Autodesk Inventor part; units mm, degrees
ref_plane "YZ Plane" through (0, 0, 0) normal (1, 0, 0) x (0, 1, 0)
ref_plane "XZ Plane" through (0, 0, 0) normal (0, 1, 0) x (-1, 0, 0)
ref_plane "XY Plane" through (0, 0, 0) normal (0, 0, 1) x (1, 0, 0)
sketch "Sketch1" plane through (0, 0, 0) normal (0, 1, 0) x (-1, 0, 0)
  line L0 (0, 0) -> (-120, 0)
  line L1 (-120, 0) -> (-120, 70)
  line L2 (-120, 70) -> (0, 70)
  line L3 (0, 70) -> (0, 0)
  dimension "d0" = 120
  dimension "d1" = 70
extrude "Extrusion1" add sketch "Sketch1" along normal blind 1
sketch "Sketch2" plane through (0, 1, 0) normal (0, 1, 0) x (1, 0, 0)
  line L0 (120, -70) -> (120, 0)
  line L1 (120, 0) -> (0, 0)
  line L2 (120, -70) -> (90, -70)
  line L3 (90, -70) -> (90, 0)
  line L4 (90, 0) -> (120, 0)
  line L5 (120, 0) -> (120, -70)
  line L6 (0, 0) -> (0, -70)
  line L7 (0, -70) -> (90, -70)
  line L8 (90, -70) -> (90, -11)
  line L9 (90, -11) -> (0, -11)
  line L10 (0, -11) -> (0, -70)
  line L11 (0, 0) -> (84, 0)
  line L12 (84, 0) -> (84, -42)
  line L13 (84, -42) -> (0, -42)
  line L14 (0, -42) -> (0, 0)
  line L15 (0, 0) -> (6, 0)
  line L16 (6, 0) -> (6, -6)
  line L17 (6, -6) -> (0, -6)
  line L18 (0, -6) -> (0, 0)
  line L19 (84, 0) -> (78, 0)
  line L20 (78, 0) -> (78, -6)
  line L21 (78, -6) -> (84, -6)
  line L22 (84, -6) -> (84, 0)
  line L23 (90, 0) -> (120, 0)
  line L24 (120, 0) -> (120, -6)
  line L25 (120, -6) -> (90, -6)
  line L26 (90, -6) -> (90, 0)
  line L27 (0, -42) -> (6, -42)
  line L28 (6, -42) -> (6, -36)
  line L29 (6, -36) -> (0, -36)
  line L30 (0, -36) -> (0, -42)
  line L31 (84, -42) -> (78, -42)
  line L32 (78, -42) -> (78, -36)
  line L33 (78, -36) -> (84, -36)
  line L34 (84, -36) -> (84, -42)
  line L35 (90, -70) -> (120, -70)
  line L36 (120, -70) -> (120, -64)
  line L37 (120, -64) -> (90, -64)
  line L38 (90, -64) -> (90, -70)
  line L39 (6, -6) -> (78, -6)
  line L40 (78, -6) -> (78, -36)
  line L41 (78, -36) -> (6, -36)
  line L42 (6, -36) -> (6, -6)
  line L43 (90, 0) -> (105, 0)
  line L44 (105, 0) -> (105, -20.5)
  line L45 (105, -20.5) -> (90, -20.5)
  line L46 (90, -20.5) -> (90, 0)
  circle A0 centre (105, -20.5) radius 6.75
  line L47 (90, -70) -> (105, -70)
  line L48 (105, -70) -> (105, -49.5)
  line L49 (105, -49.5) -> (90, -49.5)
  line L50 (90, -49.5) -> (90, -70)
  circle A1 centre (105, -49.5) radius 6.75
  point P0 (90, -64)
  point P1 (90, -6)
  point P2 (120, -6)
  point P3 (78, 0)
  point P4 (0, -36)
  point P5 (0, -42)
  point P6 (6, -11)
  point P7 (6, -36)
  point P8 (79, -29)
  point P9 (78, -11)
  dimension "d4" = 30
  dimension "d5" = 59
  dimension "d6" = 84
  dimension "d7" = 42
  dimension "d8" = 6
  dimension "d9" = 6
  dimension "d10" = 6
  dimension "d11" = 6
  dimension "d12" = 6
  dimension "d13" = 6
  dimension "d14" = 30
  dimension "d15" = 15
  dimension "d16" = 20.5
  dimension "d17" = 13.5
  dimension "d18" = 15
  dimension "d19" = 20.5
  dimension "d20" = 13.5
extrude "Extrusion2" cut sketch "Sketch2" against normal blind 1 contours A1 L49 L48 | L48 L49 A1 | A0 L45 L44 | L44 L45 A0
extrude "Extrusion3" add sketch "Sketch2" against normal blind 4 contours L2 L48 L37 L0 | L2 L3 L37 L48 | L25 L44 L1 L0 | L25 L3 L1 L44 | L6 L29 L28 L13 | L12 L21 L20 L1 | L32 L33 L12 L13 | L6 L1 L16 L17
extrude "Extrusion4" cut sketch "Sketch2" against normal blind 4 contours L42 L9 L40 L41 | L9 L42 L39 L40
sketch "Sketch5" plane through (0, 1, 0) normal (0, 1, 0) x (1, 0, 0)
  line L0 (0, 0) -> (0, -70)
  line L1 (0, 0) -> (-1, 0)
  line L2 (-1, 0) -> (-1, 1)
  line L3 (-1, 1) -> (0, 1)
  line L4 (0, 1) -> (0, 0)
  line L5 (0, -70) -> (-1, -70)
  line L6 (-1, -70) -> (-1, -71)
  line L7 (-1, -71) -> (0, -71)
  line L8 (0, -71) -> (0, -70)
  line L9 (0, -70) -> (120, -70)
  line L10 (120, -70) -> (121, -70)
  line L11 (121, -70) -> (121, -71)
  line L12 (121, -71) -> (120, -71)
  line L13 (120, -71) -> (120, -70)
  line L14 (120, -70) -> (120, 0)
  line L15 (120, 0) -> (121, 0)
  line L16 (121, 0) -> (121, 1)
  line L17 (121, 1) -> (120, 1)
  line L18 (120, 1) -> (120, 0)
  line L19 (120, 0) -> (0, 0)
  line L20 (120, 1) -> (0, 1)
  line L21 (0, 1) -> (0, 0)
  line L22 (0, 0) -> (120, 0)
  line L23 (120, 0) -> (120, 1)
  line L24 (-1, 0) -> (0, 0)
  line L25 (0, 0) -> (0, -70)
  line L26 (0, -70) -> (-1, -70)
  line L27 (-1, -70) -> (-1, 0)
  line L28 (0, -71) -> (120, -71)
  line L29 (120, -71) -> (120, -70)
  line L30 (120, -70) -> (0, -70)
  line L31 (0, -70) -> (0, -71)
  line L32 (121, -70) -> (120, -70)
  line L33 (120, -70) -> (120, 0)
  line L34 (120, 0) -> (121, 0)
  line L35 (121, 0) -> (121, -70)
  dimension "d36" = 1
  dimension "d37" = 1
  dimension "d38" = 1
  dimension "d39" = 1
  dimension "d40" = 1
  dimension "d41" = 1
  dimension "d42" = 1
  dimension "d43" = 1
extrude "Extrusion5" add sketch "Sketch5" against normal blind 26 contours L0 L5 L27 L1 | L1 L2 L3 L4 | L4 L20 L18 L19 | L8 L7 L6 L5 | L9 L13 L28 L8 | L15 L35 L10 L14 | L18 L17 L16 L15 | L10 L11 L12 L13
sketch "Sketch6" plane through (0, -25, 0) normal (0, -1, 0) x (1, 0, 0)
  line L0 (121, 71) -> (-1, 71)
  line L1 (0, 70) -> (120, 70)
  line L2 (121, 71) -> (120, 70)
  line L3 (120, 0) -> (0, 0)
  line L4 (0, 0) -> (-1, -1)
  line L5 (-0.5, -0.5) -> (120.5, -0.5)
  line L6 (120.5, -0.5) -> (120.5, 70.5)
  line L7 (120.5, 70.5) -> (-0.5, 70.5)
  line L8 (-0.5, 70.5) -> (-0.5, -0.5)
  line L9 (121, -1) -> (-1, -1)
  line L10 (121, 71) -> (-1, 71)
  line L11 (-1, 71) -> (-1, -1)
  line L12 (-1, -1) -> (121, -1)
  line L13 (121, -1) -> (121, 71)
  point P0 (121, -1)
sketch "Sketch7" plane through (0, 1, 0) normal (0, 1, 0) x (1, 0, 0)
  point P0 (0, 0)
extrude "Extrusion6" add sketch "Sketch6" along normal blind 5 contours L2 L7 L8 L4 L11 L0 | L13 L9 L4 L5 L6 L2
properties part number "carcassa"
Can you work these out from the model? Positions are in its coordinate system, mm. A direction names the side the tool comes from. Coordinates: 2 decimals unless noted, no trailing zeros. Order: outer loops, then holes, each group sorted by start corner. A loop starts at its lowest first (then second) coordinate and runs counter-clockwise, first axis right, second up.
1. If we section it at C-C (z = 20.5): Please give me the cut outline in (x, y), then the cut area to 3 significant figures.
2. Thinking about a two-plate mould opening in X: for faces 1 (the face through (74, 1, 44)), 2 (the face through (0, -12, 35)), 3 (the face through (121, -14, 34)), which applies, +X half, -X half, draft (parallel to the pull), parting line (faces both ways), or undercut?
3. I'm going to push flat-ended pins straight in: pin 1 (6.5 mm diameter, centred on x = 80.5, z = 38, fed in from -Y); pin 2 (8 mm diameter, centred on x = 69, z = 57.5, fed in from -Y). Where does each tip first touch, or does it pass through?
4. For faces 4 (the face through (59, -14, 71)), 5 (the face through (105, -3, 67)), which set-ups out of +Z, -Z, +X, -X, +Y, -Y let a thin tool reach every point of the face, with its end or its side?
5. If we section it at A-A (x = 25.5): Please give me the cut outline in (y, z).
6. If we section it at B-B (z = 49.5): Please give me the cut outline in (x, y).
7. I need wall thicknesses on line 1 (X direction, y = 0.35, z = 20.5); line 2 (X direction, y = 0.4, z = 49.5); line 3 (X direction, y = -4, z = 49.5). Which ranges of each line are inside material? Lowest first, please.
8. If we section it at D-D (x = 105): Please give me the cut outline in (y, z).
Entries:
1. outline: (-1, -30) - (-0.5, -30) - (-0.5, -25) - (0, -25) - (0, 0) - (6, 0) - (6, 1) - (-1, 1) - close; (78, 0) - (98.25, 0) - (98.25, 1) - (78, 1) - close; (111.75, 0) - (120, 0) - (120, -25) - (120.5, -25) - (120.5, -30) - (121, -30) - (121, 1) - (111.75, 1) - close
1. area: 91.5 mm2
2. face 1: draft
2. face 2: undercut
2. face 3: +X half
3. pin 1: stops at y = -3
3. pin 2: stops at y = 0
4. face 4: +Z, +X, -X, +Y, -Y
4. face 5: -Y
5. outline: (-30, -1) - (1, -1) - (1, 6) - (0, 6) - (0, 0) - (-25, 0) - (-25, -0.5) - (-30, -0.5) - close; (-30, 70.5) - (-25, 70.5) - (-25, 70) - (0, 70) - (0, 36) - (1, 36) - (1, 71) - (-30, 71) - close
6. outline: (-1, -30) - (-0.5, -30) - (-0.5, -25) - (0, -25) - (0, 0) - (98.25, 0) - (98.25, 1) - (-1, 1) - close; (111.75, 0) - (120, 0) - (120, -25) - (120.5, -25) - (120.5, -30) - (121, -30) - (121, 1) - (111.75, 1) - close
7. line 1: x = -1 to 6, 78 to 98.25, 111.75 to 121
7. line 2: x = -1 to 98.25, 111.75 to 121
7. line 3: x = -1 to 0, 120 to 121
8. outline: (-30, -1) - (1, -1) - (1, 13.75) - (0, 13.75) - (0, 6) - (-3, 6) - (-3, 0) - (-25, 0) - (-25, -0.5) - (-30, -0.5) - close; (-30, 70.5) - (-25, 70.5) - (-25, 70) - (-3, 70) - (-3, 64) - (0, 64) - (0, 56.25) - (1, 56.25) - (1, 71) - (-30, 71) - close; (0, 27.25) - (1, 27.25) - (1, 42.75) - (0, 42.75) - close
